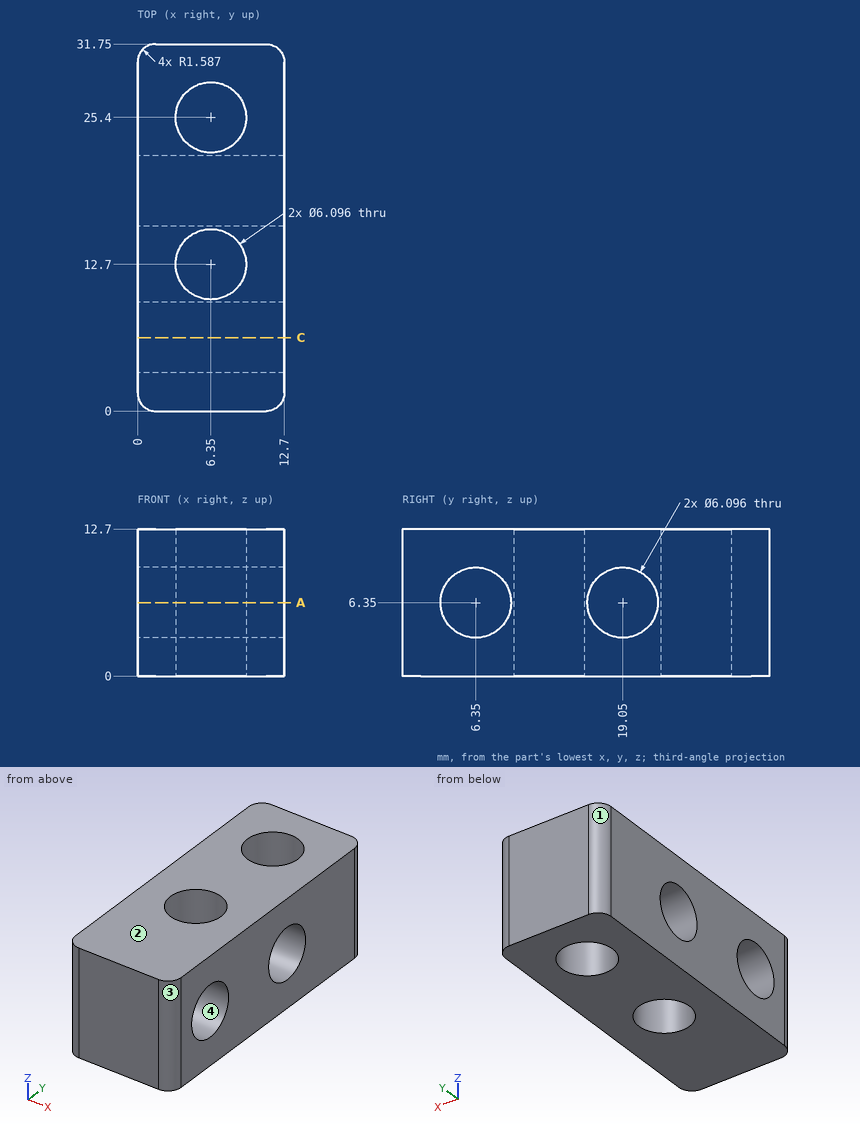
Answer from the drawing. Dimensions are ordinates in mm from the lowest x, y and z of the part. Coordinates: 2 decimals unless noted, no trailing zeros. Write each loop counter-clockwise with the first axis right and the second up, starting at its lowest first coordinate (ties: lowest second). Pieces come first, ordered by that corner, then holes. Notation, with made-up numbers: (-5.75, 47.25) -> (51.25, 47.25) arc R21 cw to (51.25, 53.25) -> close; hole circle Ø6 at (-10, 21.5). An arc over 180 degrees is marked (long way). One line per question, with ' | ' between items.
1. For a pull along Y with two mould halves and no side action, classify the marked faces 1, 2, 3 and 4 as released by +Y, released by -Y, zero draft, split by the parting line, or undercut.
Verdict:
face 1: released by +Y | face 2: zero draft | face 3: released by -Y | face 4: undercut
2. Section C-C (y = 6.35) is taken. Determine the outline of the cut face in (x, z).
Verdict:
outline: (0, 0) -> (12.7, 0) -> (12.7, 3.3) -> (0, 3.3) -> close; (0, 9.4) -> (12.7, 9.4) -> (12.7, 12.7) -> (0, 12.7) -> close
3. Straight lines are drawn through the part: line 1 (Y direction, x = 7.25, z = 2.75); line 2 (X direction, y = 25.4, z = 7.25); line 3 (Y direction, x = 7.5, z = 1.25). For each, find the intervals that lie inside material, in ascending order.
Verdict:
line 1: y = 0 to 9.79, 15.61 to 22.49, 28.31 to 31.75 | line 2: x = 0 to 3.3, 9.4 to 12.7 | line 3: y = 0 to 9.88, 15.52 to 22.58, 28.22 to 31.75
4. Section A-A (z = 6.35) is taken. State how many separate pieces and enclosed holes the cut face has, and give its area (3 significant figures).
Verdict:
separate pieces: 3 | enclosed holes: 2 | area: 188 mm^2
